from build123d import *

# Parameters (mm, degrees)
EXTRUDE1_DEPTH        = 30
FILLET1_R             = 5
M5_TAPPED_HOLE1_D     = 4.2
M6_TAPPED_HOLE1_D     = 5
M6_TAPPED_HOLE1_DEPTH = 20
M6_TAPPED_HOLE1_TIP   = 1.502151548


with BuildPart() as part:
    # Sketch1 → Extrude1 (new body)
    with BuildSketch(Plane.XY):
        with BuildLine():
            Line((-25, 30), (25, 30))
            Line((25, 30), (25, -20))
            Line((25, -20), (8.5, -20))
            Line((8.5, -20), (8.5, -11.124297731))
            ThreePointArc((8.5, -11.124297731), (0, 14), (-8.5, -11.124297731))
            Line((-8.5, -11.124297731), (-8.5, -20))
            Line((-8.5, -20), (-25, -20))
            Line((-25, -20), (-25, 30))
        make_face()
    extrude(amount=EXTRUDE1_DEPTH)

    # Fillet1
    fillet1_edges = [part.edges().sort_by_distance(p)[0] for p in [
        (-8.5, -20, 15),
        (-25, -20, 15),
        (25, -20, 15),
        (8.5, -20, 15),
        (8.5, -11.124297731, 15),
        (-8.5, -11.124297731, 15),
    ]]
    fillet(fillet1_edges, radius=FILLET1_R)

    # M5 Tapped Hole1 (through all)
    with Locations(Plane(origin=(0, 0, 0), x_dir=(-1, 0, 0), z_dir=(0, 0, -1))):
        with Locations((-13.435028843, 13.435028843), (13.435028843, 13.435028843), (19, 0), (13.435028843, -13.435028843), (-13.435028843, -13.435028843), (-19, 0)):
            Hole(M5_TAPPED_HOLE1_D / 2)

    # M6 Tapped Hole1
    with Locations(Plane(origin=(0, 30, 0), x_dir=(1, 0, 0), z_dir=(0, 1, 0))):
        with Locations((-17.5, -15), (17.5, -15)):
            Hole(M6_TAPPED_HOLE1_D / 2, depth=M6_TAPPED_HOLE1_DEPTH)
            with Locations((0, 0, -(M6_TAPPED_HOLE1_DEPTH + M6_TAPPED_HOLE1_TIP / 2))):  # 118° drill point
                Cone(0, M6_TAPPED_HOLE1_D / 2, M6_TAPPED_HOLE1_TIP, mode=Mode.SUBTRACT)


solid = part.part
Verification items for the finished model (mm, model axes). A direction names the side the tool comes from. Coordinates: 2 decimals unless noted, no trailing zeros. Write each loop counter-clockwise with the first axis right and the second up, starting at its lowest first coordinate (ties: lowest second). Pieces come first, ordered by that corner, then holes. Notation, with made-up numbers: (58.5, 84.25) - (95.5, 84.25) arc R18 ccw to (95.5, 117.25) - close; hole circle Ø3 at (25.5, -31). An arc over 180 degrees is marked (long way). Answer as a JSON object with one key per item and string values.
(1) Cross-section at C-C on x = -12.5. Record the cut outline in (y, z), plus the area to 3 significant figures.
Report:
{"outline": "(-19.9, 0) - (-15.32, 0) - (-15.32, 30) - (-19.9, 30) - close; (-11.55, 0) - (-6.3, 0) - (-6.3, 30) - (-11.55, 30) - close; (6.3, 0) - (11.55, 0) - (11.55, 30) - (6.3, 30) - close; (15.32, 0) - (30, 0) - (30, 30) - (15.32, 30) - close", "area": "893 mm^2"}
(2) Mould release check, pull along Z, two halves, no side actions. Record for faces 4 (the cylindrical face through (-23, -19, 15)), 5 (the flat face through (0, 16, 0)), 6 (the conical face through (17.18, 8.759, 14.707)), 7 (the conical face through (-17.27, 8.76, 14.63)): pulls with the +Z half, pulls with the -Z half, needs draft (parallel to the pull), parting line crosses it, or undercut.
Report:
{"face 4": "needs draft", "face 5": "pulls with the -Z half", "face 6": "undercut", "face 7": "undercut"}
(3) Cross-section at B-B on z = 9. Record the cut outline in (x, y), plus the area to 3 significant figures.
Report:
{"outline": "(-25, -15) arc R5 ccw to (-20, -20) - (-13.5, -20) arc R5 ccw to (-8.5, -15) - (-8.5, -13.37) arc R5 ccw to (-9.95, -9.85) arc R14 cw (long way) to (9.95, -9.85) arc R5 ccw to (8.5, -13.37) - (8.5, -15) arc R5 ccw to (13.5, -20) - (20, -20) arc R5 ccw to (25, -15) - (25, 30) - (-25, 30) - close; hole circle Ø4.2 at (-19, 0); hole circle Ø4.2 at (-13.44, -13.44); hole circle Ø4.2 at (-13.44, 13.44); hole circle Ø4.2 at (13.44, -13.44); hole circle Ø4.2 at (13.44, 13.44); hole circle Ø4.2 at (19, 0)", "area": "1,660 mm^2"}
(4) Cross-section at A-A on y = 0. Record the cut outline in (x, z).
Report:
{"outline": "(-25, 0) - (-21.1, 0) - (-21.1, 30) - (-25, 30) - close; (-16.9, 0) - (-14, 0) - (-14, 30) - (-16.9, 30) - close; (14, 0) - (16.9, 0) - (16.9, 30) - (14, 30) - close; (21.1, 0) - (25, 0) - (25, 30) - (21.1, 30) - close"}
(5) Gauge pin test, flat ends, axial feed: pin 1 Ø5.5 at (x, y) = (-13.44, 13.44) entering from -Z; pin 2 Ø2.5 at (x, y) = (13.44, -13.44) entering from -Z. Record the tip position at first contact, or that the pin passes through.
Report:
{"pin 1": "z = 0", "pin 2": "through"}
(6) Cross-section at D-D on y = -17. Record the cut outline in (x, z), plus the area to 3 significant figures.
Report:
{"outline": "(-24.58, 0) - (-8.92, 0) - (-8.92, 30) - (-24.58, 30) - close; (8.92, 0) - (24.58, 0) - (24.58, 30) - (8.92, 30) - close", "area": "940 mm^2"}
(7) Thickness scan on line 1 along X through (y, z) = (19.75, 15); line 2 along X through (y, z) = (-12, 23); line 3 along Y through (x, z) = (19, 5). Record the ranges inside material, lowest first.
Report:
{"line 1": "-25 to -20, -15 to 15, 20 to 25", "line 2": "-25 to -14.97, -11.9 to -8.69, 8.69 to 11.9, 14.97 to 25", "line 3": "-20 to -2.1, 2.1 to 30"}
(8) Tool access check on faces 1 (the flat face through (-25, 7, 15)), 2 (the cylindrical face through (-8.886, -11.442, 15.21)), 3 (the flat face through (8.5, -14, 15)). Record the directions out of +Z, -Z, +X, -X, +Y, -Y that give a thin tool (end or side, any length) a straight path to the whole face; none if there is none.
Report:
{"face 1": "+Z, -Z, -X, +Y, -Y", "face 2": "+Z, -Z", "face 3": "+Z, -Z, -Y"}
